```python
from build123d import *

# Parameters (mm, degrees)
EXTRUDE1_REACH           = 19.467
SKETCH11_W               = 2.8
SKETCH11_H               = 0.333333333
POINT_CUT_EXTRUDE8_DEPTH = 15.322185587
SKETCH16_R               = 2.2
CUT_EXTRUDE1_DEPTH       = 0.56


with BuildPart() as part:
    # Sketch1 → base-Revolve (revolve)
    with BuildSketch(Plane.XY, mode=Mode.PRIVATE) as base_revolve_sk:
        with BuildLine():
            Line((0, 4.25), (-0.6, 4.25))
            Line((-0.6, 4.25), (-1.087379544, 2.75))
            Line((-1.087379544, 2.75), (-3.4, 2.75))
            Line((-3.4, 2.75), (-3.4, 0))
            Line((-3.4, 0), (-2.84, 0))
            Line((-2.84, 0), (0, 0))
            Line((0, 0), (13, 0))
            Line((13, 0), (13, 2))
            Line((13, 2), (1, 2))
            Line((1, 2), (0.6, 1.6))
            Line((0.6, 1.6), (0.2, 1.6))
            ThreePointArc((0.2, 1.6), (0.058578644, 1.658578644), (0, 1.8))
            Line((0, 1.8), (0, 4.25))
        make_face()
    revolve(base_revolve_sk.sketch.rotate(Axis((0, 0, 0), (1, 0, 0)), 90), axis=Axis((0, 0, 0), (1, 0, 0)))

    # Extrude1: up to this cone (the profile starts outside it)
    extrude1_end = Plane(origin=(-3.4, 0, 0), z_dir=(1, 0, 0)).offset(1.419092291) * Cone(3.078e-06, 57.084593283, 18.547907709, align=(Align.CENTER, Align.CENTER, Align.MIN), mode=Mode.PRIVATE)
    # Sketch15 → Extrude1 (add, up to the surface)
    with BuildSketch(Plane.ZY.offset(3.4), mode=Mode.PRIVATE) as extrude1_sk1:
        Polygon((-1.58771324, 2.75), (-3.175426481, 0), (-1.58771324, -2.75), (1.58771324, -2.75), (3.175426481, 0), (1.58771324, 2.75), align=None)
    extrude1_tool1 = extrude(extrude1_sk1.sketch, amount=-EXTRUDE1_REACH, mode=Mode.PRIVATE) - extrude1_end
    add(extrude1_tool1.solids().sort_by_distance((-3.4, 0, 0))[0])

    # Sketch8 → point_Cut-Revolve1 (revolve, cut)
    with BuildSketch(Plane.XY, mode=Mode.PRIVATE) as point_cut_revolve1_sk:
        Polygon((13, 0), (13.508, 0), (13.508, 2.508), (12.194596374, 2.508), (12.194596374, 2), (13, 1.535), align=None)
    revolve(point_cut_revolve1_sk.sketch.rotate(Axis((0, 0, 0), (1, 0, 0)), 90), axis=Axis((0, 0, 0), (1, 0, 0)), mode=Mode.SUBTRACT)

    # Sketch11 → point_Cut-Extrude8 (cut, through all)
    with BuildSketch(Plane.XY):
        with Locations((11.6, -0.166666667)):
            Rectangle(SKETCH11_W, SKETCH11_H)
    extrude(amount=POINT_CUT_EXTRUDE8_DEPTH, mode=Mode.SUBTRACT)

    # Sketch16 → Cut-Extrude1 (cut)
    with BuildSketch(Plane.ZY.offset(3.4)):
        Circle(SKETCH16_R)
    extrude(amount=-CUT_EXTRUDE1_DEPTH, mode=Mode.SUBTRACT)


solid = part.part
```
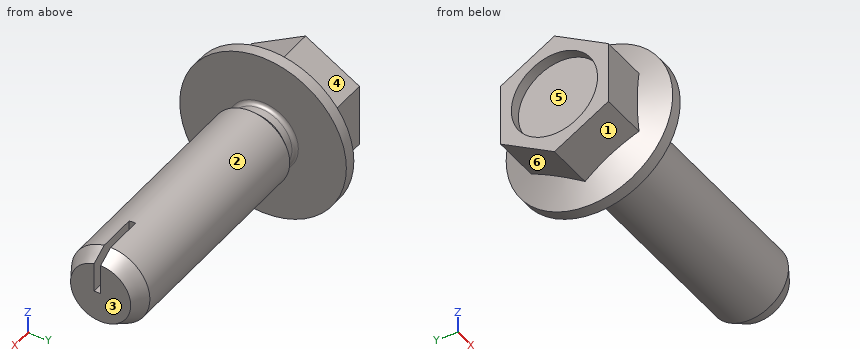
Geometry check sheet. Reference: the model listing, model coordinates, mm. Face numbers are marked on the shaded views. A direction names the side the tool comes from. Coordinates: 2 decimals unless noted, no trailing zeros. Order: outer loops, then holes, each group sorted by start corner. A loop starts at its lowest first (then second) coordinate and runs counter-clockwise, first axis right, second up.
Q1. Tool access check on the marked faces 1, 2 and 3. Record the directions out of +Z, -Z, +X, -X, +Y, -Y that give a thin tool (end or side, any length) a straight path to the whole face; none if there is none.
Reply:
face 1: -Z, -X, -Y
face 2: +X
face 3: +Z, -Z, +X, +Y, -Y
Q2. Thickness scan on probe 1 along Y at (x, z) = (-3.1, 0); probe 2 along X at (y, z) = (2, -1.5); probe 3 along X at (y, z) = (0.75, 1.25). Record the ranges inside material, lowest first.
Reply:
probe 1: y = -2.75 to -2.2, 2.2 to 2.75
probe 2: x = -3.4 to 0
probe 3: x = -2.84 to 13
Q3. Draft check along Z on the marked faces 4, 5 and 6. Enter one of: released by +Z, released by -Z, zero draft, split by the parting line, or undercut.
Reply:
face 4: released by +Z
face 5: undercut
face 6: released by -Z
Q4. Depth check by flat-ended pin: pin 1 Ø5 at (y, z) = (0, -0.5) entering from -X; pin 2 Ø5 at (x, y) = (8, 2) entering from -Z; pin 3 Ø1.6 at (x, z) = (11.5, 1.5) entering from +Y; pin 4 Ø2 at (x, z) = (-3, 0.5) entering from -Y. Enter the tip coordinate at first touch or a pass-through.
Reply:
pin 1: stops at x = -3.4
pin 2: stops at z = -2
pin 3: stops at y = 1.87
pin 4: stops at y = -2.75
Q5. Sectioned sample at A-A on x = 2. Record the cut outline in (y, z), and give its area (3 significant figures).
Reply:
outline: circle Ø4 at (0, 0)
area: 12.6 mm2
